Source: CAD feature listing. Evaluate the final solid. Frame: model axes, mm. A direction names the side the tool comes from. Round coordinates to 2 decimals unless told otherwise and drop trailing zeros. Write each loop counter-clockwise with the first axis right and the second up, starting at its lowest first coordinate (ties: lowest second). Pieces come first, ordered by that corner, then holes. Notation, with made-up numbers: (24.5, 23) -> (72.5, 23) arc R20 cw to (72.5, 42) -> close; hole circle Ø7 at (13, -26). An arc over 180 degrees is marked (long way). Put each result on its own line as item: value.
```python
from build123d import *

# Parameters (mm, degrees)
SKETCH1_W               = 239
SKETCH1_H               = 180
SKETCH1_R               = 1.75
BOSS_EXTRUDE1_DEPTH     = 10
SKETCH2_W               = 20
SKETCH2_H               = 28
BOSS_EXTRUDE2_DEPTH     = 23
SKETCH3_R               = 7.6
CUT_EXTRUDE1_DEPTH      = 219.561776164
FILLET1_R               = 10
FILLET2_R               = 10
CUT_EXTRUDE2_DEPTH      = 20
SKETCH5_W               = 104.5
SKETCH5_H               = 50
CUT_EXTRUDE3_DEPTH      = 20
FILLET3_R               = 15
FILLET4_R               = 15
CUT_EXTRUDE4_DEPTH      = 3
SKETCH7_W               = 1
SKETCH7_H               = 35.181003967
SKETCH7_H_2             = 30.639156463
SKETCH7_H_3             = 31.227118238
CUT_EXTRUDE_THIN1_DEPTH = 21


with BuildPart() as part:
    # Sketch1 → Boss-Extrude1 (new body)
    with BuildSketch(Plane(origin=(0, 0, 0), x_dir=(1, 0, 0), z_dir=(0, 1, 0))):
        Rectangle(SKETCH1_W, SKETCH1_H)
        with Locations(Location((104.5, 0, 0), (0, 0, 270))):
            Circle(SKETCH1_R, mode=Mode.SUBTRACT)
        with Locations(Location((-104.5, 75, 0), (0, 0, 270))):
            Circle(SKETCH1_R, mode=Mode.SUBTRACT)
        with Locations(Location((-104.5, -75, 0), (0, 0, 270))):
            Circle(SKETCH1_R, mode=Mode.SUBTRACT)
    extrude(amount=BOSS_EXTRUDE1_DEPTH)

    # Sketch2 → Boss-Extrude2 (add)
    with BuildSketch(Plane(origin=(0, 10, 0), x_dir=(1, 0, 0), z_dir=(0, 1, 0))):
        with Locations((-80, 76)):
            Rectangle(SKETCH2_W, SKETCH2_H)
        with Locations((-80, -76)):
            Rectangle(SKETCH2_W, SKETCH2_H)
        with Locations((80, 0)):
            Rectangle(SKETCH2_W, SKETCH2_H)
    extrude(amount=BOSS_EXTRUDE2_DEPTH)

    # Sketch3 → Cut-Extrude1 (cut, symmetric)
    with BuildSketch(Plane(origin=(0, 0, -90), x_dir=(-1, 0, 0), z_dir=(0, 0, -1))):
        with Locations((80, 23.4)):
            Circle(SKETCH3_R)
    cut_extrude1 = extrude(amount=CUT_EXTRUDE1_DEPTH, both=True, mode=Mode.SUBTRACT)

    # Fillet1
    fillet1_edges = [part.edges().sort_by_distance(p)[0] for p in [
        (90, 33, 0),
        (70, 33, 0),
        (-90, 33, 76),
        (-70, 33, 76),
        (-70, 33, -76),
        (-90, 33, -76),
    ]]
    fillet(fillet1_edges, radius=FILLET1_R - 0.0001)  # a hair under: the kernel refuses the full size

    # Mirror1: Cut-Extrude1 across plane
    add(cut_extrude1.mirror(Plane(origin=(0, 0, 0), x_dir=(0, 0, 1), z_dir=(1, 0, 0))), mode=Mode.SUBTRACT)

    # Fillet2
    fillet2_edges = [part.edges().sort_by_distance(p)[0] for p in [
        (-70, 10, -76),
        (-90, 10, -76),
        (-70, 10, 76),
        (-90, 10, 76),
        (70, 10, 0),
        (90, 10, 0),
    ]]
    fillet(fillet2_edges, radius=FILLET2_R)

    # Sketch4 → Cut-Extrude2 (cut)
    with BuildSketch(Plane(origin=(0, 10, 0), x_dir=(1, 0, 0), z_dir=(0, 1, 0))):
        with BuildLine():
            Line((-35, 62), (-25, 62))
            ThreePointArc((-25, 62), (-17.928932188, 59.071067812), (-15, 52))
            Line((-15, 52), (-15, -52))
            ThreePointArc((-15, -52), (-17.928932188, -59.071067812), (-25, -62))
            Line((-25, -62), (-35, -62))
            ThreePointArc((-35, -62), (-42.071067812, -59.071067812), (-45, -52))
            Line((-45, -52), (-45, 52))
            ThreePointArc((-45, 52), (-42.071067812, 59.071067812), (-35, 62))
        make_face()
    extrude(amount=-CUT_EXTRUDE2_DEPTH, mode=Mode.SUBTRACT)

    # Sketch5 → Cut-Extrude3 (cut)
    with BuildSketch(Plane(origin=(0, 10, 0), x_dir=(1, 0, 0), z_dir=(0, 1, 0))):
        with Locations((67.25, 65)):
            Rectangle(SKETCH5_W, SKETCH5_H)
    cut_extrude3 = extrude(amount=-CUT_EXTRUDE3_DEPTH, mode=Mode.SUBTRACT)

    # Fillet3
    fillet3_edges = [part.edges().sort_by_distance(p)[0] for p in [
        (15, 5, -90),
        (119.5, 5, -40),
        (15, 5, -40),
        (-119.5, 5, -90),
    ]]
    fillet(fillet3_edges, radius=FILLET3_R)

    # Mirror2: Cut-Extrude3 across plane
    add(cut_extrude3.mirror(Plane.XY), mode=Mode.SUBTRACT)

    # Fillet4
    fillet4_edges = [part.edges().sort_by_distance(p)[0] for p in [
        (15, 5, 90),
        (119.5, 5, 40),
        (15, 5, 40),
        (-119.5, 5, 90),
    ]]
    fillet(fillet4_edges, radius=FILLET4_R)

    # Sketch6 → Cut-Extrude4 (cut)
    with BuildSketch(Plane(origin=(0, 10, 0), x_dir=(1, 0, 0), z_dir=(0, 1, 0))):
        Polygon((-107.964101615, -75), (-106.232050808, -78), (-102.767949192, -78), (-101.035898385, -75), (-102.767949192, -72), (-106.232050808, -72), align=None)
        Polygon((-107.964101615, 75), (-106.232050808, 72), (-102.767949192, 72), (-101.035898385, 75), (-102.767949192, 78), (-106.232050808, 78), align=None)
        Polygon((107.964101615, 0), (106.232050808, 3), (102.767949192, 3), (101.035898385, 0), (102.767949192, -3), (106.232050808, -3), align=None)
    extrude(amount=-CUT_EXTRUDE4_DEPTH, mode=Mode.SUBTRACT)

    # Sketch7 → Cut-Extrude-Thin1 (cut)
    with BuildSketch(Plane(origin=(0, 25, 0), x_dir=(1, 0, 0), z_dir=(0, 1, 0))):
        with Locations((-80, -79.590501984)):
            Rectangle(SKETCH7_W, SKETCH7_H)
        with Locations((-80, 74.680421768)):
            Rectangle(SKETCH7_W, SKETCH7_H_2)
        with Locations((80, -1.613559119)):
            Rectangle(SKETCH7_W, SKETCH7_H_3)
    extrude(amount=CUT_EXTRUDE_THIN1_DEPTH, mode=Mode.SUBTRACT)


solid = part.part
```
Q1. Draft query along X for faces 1 (the flat face through (-103, 7, -76.4)), 2 (the cylindrical face through (-93.01, 12.85, -76.2)), 3 (the flat face through (-80, 15, 62)). Return one class per face: +X half, -X half, draft (parallel to the pull), parting line (faces both ways), or undercut.
Ans:
face 1: undercut
face 2: -X half
face 3: draft
Q2. Reachability of faces 4 (the flat face through (-30, 5, 62)), 5 (the flat face through (67, 5, 40)), 6 (the cylindrical face through (-66.99, 12.85, 75.8)), 7 (the flat face through (15, 5, -65)), 8 (the flat face through (80, 15, 14)) from +Z, -Z, +X, -X, +Y, -Y: full face, straight path, thin tool, end or side. Return the list, or none.
Ans:
face 4: +Y, -Y
face 5: +Z, +X, +Y, -Y
face 6: +Z, -Z, +X, +Y
face 7: -Z, +X, +Y, -Y
face 8: +Z, +X, -X, +Y
Q3. Cut plane A-A on y = 27. Output: boundary loops of the cut face in (x, z).
Ans:
outline: (-89.17, -90) -> (-86.69, -90) -> (-86.69, -62) -> (-89.17, -62) -> close; (-89.17, 62) -> (-86.69, 62) -> (-86.69, 90) -> (-89.17, 90) -> close; (-73.31, -90) -> (-70.83, -90) -> (-70.83, -62) -> (-73.31, -62) -> close; (-73.31, 62) -> (-70.83, 62) -> (-70.83, 90) -> (-73.31, 90) -> close; (70.83, -14) -> (73.31, -14) -> (73.31, 14) -> (70.83, 14) -> close; (86.69, -14) -> (89.17, -14) -> (89.17, 14) -> (86.69, 14) -> close
Q4. Cut plane C-C on x = -84.5. Output: boundary loops of the cut face in (y, z).
Ans:
outline: (0, -90) -> (17.28, -90) -> (17.28, -62) -> (10, -62) -> (10, 62) -> (17.28, 62) -> (17.28, 90) -> (0, 90) -> close; (29.52, -90) -> (31.93, -90) -> (31.93, -62) -> (29.52, -62) -> close; (29.52, 62) -> (31.93, 62) -> (31.93, 90) -> (29.52, 90) -> close
Q5. Pin query (flat end, axial travel): pin 1 (1.5 mm diameter, centred on y = 22, z = -82.5, fed in from +X); pin 2 (1 mm diameter, centred on y = 32, z = 77.5, fed in from +X); pin 3 (3 mm diameter, centred on x = 61, y = 3, fed in from -Z); pin 4 (2 mm diameter, centred on x = -63.5, z = 38, fed in from -Y). Return the tip coordinate at first contact, or that it passes through.
Ans:
pin 1: stops at x = -70
pin 2: stops at x = -74.73
pin 3: stops at z = -40
pin 4: stops at y = 0
Q6. Cut plane B-B on z = -45. Output: boundary loops of the cut face in (x, y).
Ans:
outline: (-119.5, 0) -> (-45, 0) -> (-45, 10) -> (-119.5, 10) -> close; (-15, 0) -> (18.82, 0) -> (18.82, 10) -> (-15, 10) -> close
Q7. Material intervals for line 1 (X direction, y = 23, z = -79); line 2 (X direction, y = 2, z = -75); line 3 (Z direction, x = -27, y = 7), sorted ascending. Write a range as [from, to].
Ans:
line 1: x = [-90, -87.59], [-72.41, -70]
line 2: x = [-119.5, -106.25], [-102.75, 15]
line 3: z = [-90, -62], [62, 90]
